Input: part model. Units: mm. Frame: model coordinates. A direction names the side the tool comes from. Coordinates: 2 decimals unless noted, no trailing zeros. Order: outer loops, then holes, each group sorted by start corner. A loop starts at its lowest first (then second) coordinate and runs counter-clockwise, first axis right, second up. Notation, with made-up numbers: M 41.25,-15 L 49.25,-15 A15 ccw 49.25,5 Z; hole C 2,13 d5. An arc over 180 degrees is marked long. One line per item, written item: value.
Autodesk Inventor part; units mm, degrees
ref_plane "Start Plane" through (0, 0, 12.7) normal (0, 0, 1) x (1, 0, 0)
ref_plane "End Plane" through (0, 0, 622.3) normal (0, 0, 1) x (1, 0, 0)
ref_plane "Work Plane6" through (0, -38.1, 622.3) normal (0, 0, 1) x (1, 0, 0)
ref_plane "Start Plane" through (0, 0, 12.7) normal (0, 0, 1) x (1, 0, 0)
ref_plane "End Plane" through (0, 0, 622.3) normal (0, 0, 1) x (1, 0, 0)
sketch "Sketch" plane through (0, 0, 0) normal (0, 0, 1) x (1, 0, 0)
  line L0 (-12.7, -38.1) -> (12.7, -38.1)
  line L1 (12.7, -38.1) -> (12.7, 38.1)
  line L2 (12.7, 38.1) -> (-12.7, 38.1)
  line L3 (-12.7, 38.1) -> (-12.7, -38.1)
  line L4 (-12.7, -38.1) -> (12.7, 38.1) construction
  line L5 (12.7, -38.1) -> (-12.7, 38.1) construction
  line L6 (-9.525, -34.925) -> (9.525, -34.925)
  line L7 (9.525, -34.925) -> (9.525, 34.925)
  line L8 (9.525, 34.925) -> (-9.525, 34.925)
  line L9 (-9.525, 34.925) -> (-9.525, -34.925)
  line L10 (-9.525, -34.925) -> (9.525, 34.925) construction
  line L11 (9.525, -34.925) -> (-9.525, 34.925) construction
  point P0 (0, 0)
  dimension "d0" = 25.4
  dimension "d1" = 76.2
  dimension "d2" = 3.175
  dimension "d3" = 3.175
extrude "Body" add sketch "Sketch" along normal up to surface (609.6 mm away) from surface at 12.7
sketch "Sketch6" plane through (0, 0, 0) normal (0, 0, 1) x (1, 0, 0)
  line L0 (0, 0) -> (10, 0)
ref_plane "Work Plane5" through (0, 0, 0) normal (0, -1, 0) x (1, 0, 0)
sketch "Sketch7" plane through (0, 0, 0) normal (0, -1, 0) x (1, 0, 0)
  line L0 (-2, 12.7) -> (12, 12.7)
  line L1 (-2, 622.3) -> (12, 622.3)
  dimension "d11" = 609.6
ref_plane "Work Plane6" through (0, -38.1, 622.3) normal (0, 0, 1) x (1, 0, 0)
split "Split1" plane through (0, -38.1, 622.3) removes the side toward (0, 0, 1)
ref_plane "Work Plane7" through (711.2, -38.1, 12.7) normal (0, 0, -1) x (-1, 0, 0)
split "Split2" plane through (711.2, -38.1, 12.7) removes the side toward (0, 0, -1)
equation "\"d0\" = Width"
equation "\"d1\" = Height"
equation "\"d2\" = Thickness"
equation "\"d3\" = Thickness"
equation "\"Height\" = 76.2"
equation "\"Width\" = 25.4"
equation "\"Thickness\" = 3.175"
equation "\"BaseLength\" = 635"
equation "\"G_OFFSET_START\" = -12.7"
equation "\"G_OFFSET_END\" = -12.7"
equation "\"d6\" = -G_OFFSET_START"
equation "\"d7\" = BaseLength + G_OFFSET_END"
equation "\"G_L\" = d11"
properties part number "AL RECT TUBE 3 x 1 x 0.125" material "Aluminum 6061"
(1) Draft query along X for faces 1 (the flat face through (-12.7, 1, 313)), 2 (the flat face through (0, -34.925, 313)), 3 (the flat face through (0, 38.1, 313)). Return one class per face: released by +X, released by -X, zero draft, split by the parting line, or undercut.
Data:
face 1: released by -X
face 2: undercut
face 3: zero draft
(2) Access query for faces 4 (the flat face through (12.7, -1, 313)), 5 (the flat face through (-9.525, 0, 313)). Directions: +Z, -Z, +X, -X, +Y, -Y. A direction counts if a zero-diameter tool reaches every point of the face in a straight line with its end or side. Return the directions, or none.
Data:
face 4: +Z, -Z, +X, +Y, -Y
face 5: +Z, -Z
(3) Cut plane B-B on z = 424. Output: boundary loops of the cut face in (x, y) (3 decimals), plus the area to 3 significant figures.
Data:
outline: M -12.7,-38.1 L 12.7,-38.1 L 12.7,38.1 L -12.7,38.1 Z; hole M -9.525,-34.925 L 9.525,-34.925 L 9.525,34.925 L -9.525,34.925 Z
area: 605 mm2
(4) Cut plane A-A on x = -5.25. Output: boundary loops of the cut face in (y, z) (3 decimals).
Data:
outline: M -38.1,12.7 L -34.925,12.7 L -34.925,622.3 L -38.1,622.3 Z; M 34.925,12.7 L 38.1,12.7 L 38.1,622.3 L 34.925,622.3 Z
(5) Cut plane C-C on y = 18.5. Output: boundary loops of the cut face in (x, z) (3 decimals), plus the area to 3 significant figures.
Data:
outline: M -12.7,12.7 L -9.525,12.7 L -9.525,622.3 L -12.7,622.3 Z; M 9.525,12.7 L 12.7,12.7 L 12.7,622.3 L 9.525,622.3 Z
area: 3,870 mm2
(6) Ray query, line 1 (Y direction, x = -1.25, z = 96.5) (3 decimals); line 2 (X direction, y = -17, z = 566) (3 decimals). Return the intervals inside material, ascending. Write a range as from..to.
Data:
line 1: y = -38.1..-34.925, 34.925..38.1
line 2: x = -12.7..-9.525, 9.525..12.7
